CAD build for the part. Positions are in the model's coordinates, mm. A direction names the side the tool comes from. Give positions to 0.01 mm unless a question says otherwise; leave off trailing zeros. Order: outer loops, then holes, each group sorted by start corner. A loop starts at its lowest first (then second) coordinate and runs counter-clockwise, first axis right, second up.
Autodesk Inventor part; units mm, degrees
ref_plane "YZ Plane" through (0, 0, 0) normal (1, 0, 0) x (0, 1, 0)
ref_plane "XZ Plane" through (0, 0, 0) normal (0, 1, 0) x (-1, 0, 0)
ref_plane "XY Plane" through (0, 0, 0) normal (0, 0, 1) x (1, 0, 0)
sketch "Sketch1" plane through (0, 0, 0) normal (0, 0, 1) x (1, 0, 0)
  line L0 (-39.5, 0) -> (39.5, 0)
  line L1 (-39.5, 0) -> (-39.5, 40)
  arc A0 (39.5, 40) -> (-39.5, 40) centre (0, 40) ccw
  line L2 (39.5, 40) -> (39.5, 0)
  circle A1 centre (0, 40) radius 17.5
  point P0 (0, 0)
  point P1 (0, 0)
  dimension "d6" = 35
  dimension "d7" = 22
  dimension "d8" = 40
extrude "Plate1" add sketch "Sketch1" along normal blind 2
sketch "Sketch3" plane through (39.5, 2, 0) normal (0, -1, 0) x (1, 0, 0)
  line L0 (-79, 0) -> (0, 0)
  line L1 (0, 0) -> (0, 50)
  line L2 (0, 50) -> (-79, 50)
  line L3 (-79, 50) -> (-79, 0)
edge flange "Flange1" height 50 angle 90 thickness 2 bend radius 2.75 thickness toward (0, -1, 0) relief round relief width 2 relief depth 1 edges at (0, 0, 2) wall of the first edge with corners at (-39.5, 2, 0) (39.5, 2, 0) (39.5, 2, 50) (-39.5, 2, 50)
bend "Bend1"
corner "Corner1"
fillet "Corner Round1" radius 6 2 edges at (39.5, 1, 50) (-39.5, 1, 50)
equation "\"d2\" = Thickness"
equation "\"d9\" = BendReliefWidth"
equation "\"d10\" = BendReliefDepth"
equation "\"d11\" = MinimumRemnant"
equation "\"d12\" = TransitionRadius"
equation "\"d15\" = BendRadius"
equation "\"d16\" = CornerReliefSize"
equation "\"d17\" = GapSize"
equation "\"d18\" = JacobiRadiusSize"
equation "\"BendReliefWidth\" = Thickness"
equation "\"BendReliefDepth\" = 0.5 * Thickness"
equation "\"CornerReliefSize\" = 4 * Thickness"
equation "\"MinimumRemnant\" = 2 * Thickness"
equation "\"TransitionRadius\" = BendRadius"
equation "\"JacobiRadiusSize\" = BendRadius"
equation "\"GapSize\" = Thickness"
properties part number "D-ring 11" material "Stainless Steel"
Item 1: Slice it at A-A (y = 26). Give the cut face in (x, z).
Item 2: Drop flat-ended pins along their axis: pin 1 Ø6 at (x, z) = (20.5, 24.5) entering from +Y; pin 2 Ø8 at (x, y) = (-2, 61.5) entering from -Z. Give the stop position or say it passes through.
Item 3: Wall check: L1, parallel to Z at x = -31.5, y = 37.5; L2, parallel to Y at x = 0, z = 1. Give the ranges that are in metal, low to high.
Item 4: Tool access for faces 1 (the face through (1, 2, 27)), 2 (the face through (-18, 43, 0)): list every direction of +Z, -Z, +X, -X, +Y, -Y with a clear straight run to the whole face (end or side of a thin tool).
Item 5: Slice it at D-D (y = 42.5). Give the cut face in (x, z).
Item 6: Slice it at B-B (x = 0). Give the cut face in (y, z), and give its area (3 significant figures).
Item 7: Slice it at C-C (x = -23). Give the cut face in (y, z).
A:
1. outline: (-39.5, 0) - (-10.5, 0) - (-10.5, 2) - (-39.5, 2) - close; (10.5, 0) - (39.5, 0) - (39.5, 2) - (10.5, 2) - close
2. pin 1: stops at y = 2
2. pin 2: stops at z = 0
3. L1: z = 0 to 2
3. L2: y = 1.83 to 22.5, 57.5 to 79.5
4. face 1: +Z, +X, -X, +Y
4. face 2: -Z, +X, -X, +Y, -Y
5. outline: (-39.42, 0) - (-17.32, 0) - (-17.32, 2) - (-39.42, 2) - close; (17.32, 0) - (39.42, 0) - (39.42, 2) - (17.32, 2) - close
6. outline: (0, 4.75) arc R4.75 ccw to (4.75, 0) - (22.5, 0) - (22.5, 2) - (4.75, 2) arc R2.75 cw to (2, 4.75) - (2, 50) - (0, 50) - close; (57.5, 0) - (79.5, 0) - (79.5, 2) - (57.5, 2) - close
6. area: 182 mm2
7. outline: (0, 4.75) arc R4.75 ccw to (4.75, 0) - (72.11, 0) - (72.11, 2) - (4.75, 2) arc R2.75 cw to (2, 4.75) - (2, 50) - (0, 50) - close
